Build history of the part. All positions in model axes, mm. A direction names the side the tool comes from. Coordinates: 2 decimals unless noted, no trailing zeros. Order: outer loops, then holes, each group sorted by start corner. A loop starts at its lowest first (then second) coordinate and runs counter-clockwise, first axis right, second up. Notation, with made-up numbers: (24.25, 78) - (52.25, 78) arc R12 cw to (52.25, 88) - close; hole circle Ø1 at (-40, -9). An arc over 180 degrees is marked (long way). Write each question's results on one line, items separated by ' | '.
from build123d import *

# Parameters (mm, degrees)
SKETCH1_W           = 40
SKETCH1_H           = 40
SKETCH1_W_2         = 34
SKETCH1_H_2         = 34
BOSS_EXTRUDE1_DEPTH = 489.5
FILLET1_R           = 1
FILLET2_R           = 3
SKETCH2_W           = 40
SKETCH2_H           = 115
SKETCH2_R           = 4.5
BOSS_EXTRUDE2_DEPTH = 3
FILLET3_R           = 3
FILLET4_R           = 3


with BuildPart() as part:
    # Sketch1 → Boss-Extrude1 (new body)
    with BuildSketch(Plane(origin=(0, 0, 0), x_dir=(0, 0, -1), z_dir=(1, 0, 0))):
        Rectangle(SKETCH1_W, SKETCH1_H)
        Rectangle(SKETCH1_W_2, SKETCH1_H_2, mode=Mode.SUBTRACT)
    extrude(amount=BOSS_EXTRUDE1_DEPTH)

    # Fillet1
    fillet1_edges = [part.edges().sort_by_distance(p)[0] for p in [
        (244.75, -17, -17),
        (244.75, 17, -17),
        (244.75, 17, 17),
        (244.75, -17, 17),
    ]]
    fillet(fillet1_edges, radius=FILLET1_R)

    # Fillet2
    fillet2_edges = [part.edges().sort_by_distance(p)[0] for p in [
        (244.75, -20, -20),
        (244.75, -20, 20),
        (244.75, 20, 20),
        (244.75, 20, -20),
    ]]
    fillet(fillet2_edges, radius=FILLET2_R)

    # Sketch2 → Boss-Extrude2 (add)
    with BuildSketch(Plane(origin=(489.5, 0, 0), x_dir=(0, 0, -1), z_dir=(1, 0, 0))):
        Rectangle(SKETCH2_W, SKETCH2_H)
        Circle(SKETCH2_R, mode=Mode.SUBTRACT)
        with Locations((0, -37.5)):
            Circle(SKETCH2_R, mode=Mode.SUBTRACT)
        with Locations((0, 37.5)):
            Circle(SKETCH2_R, mode=Mode.SUBTRACT)
    extrude(amount=BOSS_EXTRUDE2_DEPTH)

    # Fillet3
    # the kernel refuses this fillet: 3 mm, written as the material it adds along each edge
    with BuildSketch(Plane(origin=(489.5, -20, 17), x_dir=(0, -1, 0), z_dir=(0, 0, -1)), Plane(origin=(489.5, 20, -17), x_dir=(0, 1, 0), z_dir=(0, 0, 1))) as fillet3_piece_1:
        with BuildLine():
            CenterArc((FILLET3_R, FILLET3_R), FILLET3_R, 180, 90)
            Line((0, FILLET3_R), (0, 0))
            Line((0, 0), (FILLET3_R, 0))
        make_face()
    extrude(amount=34)
    with BuildSketch(Plane(origin=(489.5, 17, 17), x_dir=(0, 1, 0), z_dir=(0, 0, -1))) as fillet3_piece_2_section:
        with BuildLine():
            CenterArc((3 + FILLET3_R, -FILLET3_R), FILLET3_R, 90, 90)
            Line((3, -FILLET3_R), (3, 0))
            Line((3, 0), (3 + FILLET3_R, 0))
        make_face()
    fillet3_piece_2 = revolve(axis=Axis((489.5, 17, 17), (1, 0, 0)), revolution_arc=233.296989237, mode=Mode.PRIVATE)
    fillet3_piece_2 = split(fillet3_piece_2, bisect_by=Plane(origin=(488.998099396, 20.659325751, 20), z_dir=(0, 0, -1)), keep=Keep.TOP, mode=Mode.PRIVATE)
    fillet3_piece_2 = split(fillet3_piece_2, bisect_by=Plane(origin=(488.998099396, 20.659325751, 17), z_dir=(0, 0, 1)), keep=Keep.TOP, mode=Mode.PRIVATE)
    add(fillet3_piece_2)
    with BuildSketch(Plane(origin=(489.5, 17, -17), x_dir=(0, -0.5976672776328276, 0.8017442392976482), z_dir=(0, 0.8017442392976482, 0.5976672776328276))) as fillet3_piece_3_section:
        with BuildLine():
            CenterArc((3 + FILLET3_R, -FILLET3_R), FILLET3_R, 90, 90)
            Line((3, -FILLET3_R), (3, 0))
            Line((3, 0), (3 + FILLET3_R, 0))
        make_face()
    fillet3_piece_3 = revolve(axis=Axis((489.5, 17, -17), (1, 0, 0)), revolution_arc=233.296989237, mode=Mode.PRIVATE)
    fillet3_piece_3 = split(fillet3_piece_3, bisect_by=Plane(origin=(488.565115083, 19.249816872, -20), z_dir=(0, 0, 1)), keep=Keep.TOP, mode=Mode.PRIVATE)
    fillet3_piece_3 = split(fillet3_piece_3, bisect_by=Plane(origin=(488.565115083, 19.249816872, -17), z_dir=(0, 0, -1)), keep=Keep.TOP, mode=Mode.PRIVATE)
    add(fillet3_piece_3)
    with BuildSketch(Plane(origin=(489.5, -17, -17), x_dir=(0, -1, 0), z_dir=(0, 0, 1))) as fillet3_piece_4_section:
        with BuildLine():
            CenterArc((3 + FILLET3_R, -FILLET3_R), FILLET3_R, 90, 90)
            Line((3, -FILLET3_R), (3, 0))
            Line((3, 0), (3 + FILLET3_R, 0))
        make_face()
    fillet3_piece_4 = revolve(axis=Axis((489.5, -17, -17), (1, 0, 0)), revolution_arc=233.296989237, mode=Mode.PRIVATE)
    fillet3_piece_4 = split(fillet3_piece_4, bisect_by=Plane(origin=(488.998099396, -20.659325751, -20), z_dir=(0, 0, 1)), keep=Keep.TOP, mode=Mode.PRIVATE)
    fillet3_piece_4 = split(fillet3_piece_4, bisect_by=Plane(origin=(488.998099396, -20.659325751, -17), z_dir=(0, 0, -1)), keep=Keep.TOP, mode=Mode.PRIVATE)
    add(fillet3_piece_4)
    with BuildSketch(Plane(origin=(489.5, -17, 17), x_dir=(0, -1, 0), z_dir=(0, 0, -1))) as fillet3_piece_5_section:
        with BuildLine():
            CenterArc((3 + FILLET3_R, FILLET3_R), FILLET3_R, 180, 90)
            Line((3, FILLET3_R), (3, 0))
            Line((3, 0), (3 + FILLET3_R, 0))
        make_face()
    fillet3_piece_5 = revolve(axis=Axis((489.5, -17, 17), (-1, 0, 0)), revolution_arc=233.296989237, mode=Mode.PRIVATE)
    fillet3_piece_5 = split(fillet3_piece_5, bisect_by=Plane(origin=(488.998099366, -20.659325736, 20), z_dir=(0, 0, -1)), keep=Keep.TOP, mode=Mode.PRIVATE)
    fillet3_piece_5 = split(fillet3_piece_5, bisect_by=Plane(origin=(488.998099366, -20.659325736, 17), z_dir=(0, 0, 1)), keep=Keep.TOP, mode=Mode.PRIVATE)
    add(fillet3_piece_5)

    # Fillet4
    fillet4_edges = [part.edges().sort_by_distance(p)[0] for p in [
        (491, -57.5, -20),
        (491, 57.5, -20),
        (491, 57.5, 20),
        (491, -57.5, 20),
    ]]
    fillet(fillet4_edges, radius=FILLET4_R)

    # Mirror1: part across plane


with BuildPart() as part_1:
    add(part.part)
    add(part.part.mirror(Plane(origin=(0, 0, 0), x_dir=(0, 0, 1), z_dir=(1, 0, 0))))


solid = part_1.part
1. Probe line 1 (Y direction, x = -491.05, z = 0); line 2 (X direction, y = 15.5, z = -16.5); line 3 (Y direction, x = 243, z = -7.5). List the from-to ranges inside material, lowest first.
Solved:
line 1: y = -57.5 to -42, -33 to -4.5, 4.5 to 33, 42 to 57.5 | line 2: x = -492.5 to -489.5, 489.5 to 492.5 | line 3: y = -20 to -17, 17 to 20
2. Two-plate mould, pull along Y, no slides. Class faces 1 (the face through (7, 17, 0)), 2 (the face through (-489.5, -44, 0)), 3 (the face through (7, 20, 0)): +Y half, -Y half, draft (parallel to the pull), parting line (faces both ways), or undercut.
Solved:
face 1: undercut | face 2: draft | face 3: +Y half
3. Band-saw the part on A-A on x = 96.5. Give the cut face in (y, z).
Solved:
outline: (-20, -17) arc R3 ccw to (-17, -20) - (17, -20) arc R3 ccw to (20, -17) - (20, 17) arc R3 ccw to (17, 20) - (-17, 20) arc R3 ccw to (-20, 17) - close; hole (-17, -16) arc R1 ccw to (-16, -17) - (16, -17) arc R1 ccw to (17, -16) - (17, 16) arc R1 ccw to (16, 17) - (-16, 17) arc R1 ccw to (-17, 16) - close
4. Drop flat-ended pins along their axis: pin 1 Ø10.5 at (y, z) = (0, 0) entering from +X; pin 2 Ø4 at (x, y) = (229.5, -23.5) entering from -Z; pin 3 Ø10 at (x, z) = (181, 4) entering from -Y; pin 4 Ø16 at (x, z) = (146, 6) entering from +Y. Give the stop position or say it passes through.
Solved:
pin 1: stops at x = 492.5 | pin 2: passes through | pin 3: stops at y = -20 | pin 4: stops at y = 20
5. Tool access for faces 4 (the face through (7, -20, 0)), 5 (the face through (-492.5, 1, 5)), 6 (the face through (7, -17, 0)), 7 (the face through (489.5, 44, 0)): list every direction of +Z, -Z, +X, -X, +Y, -Y with a clear straight run to the whole face (end or side of a thin tool).
Solved:
face 4: +Z, -Z, -Y | face 5: +Z, -Z, -X, +Y, -Y | face 6: none | face 7: +Z, -Z, +Y
